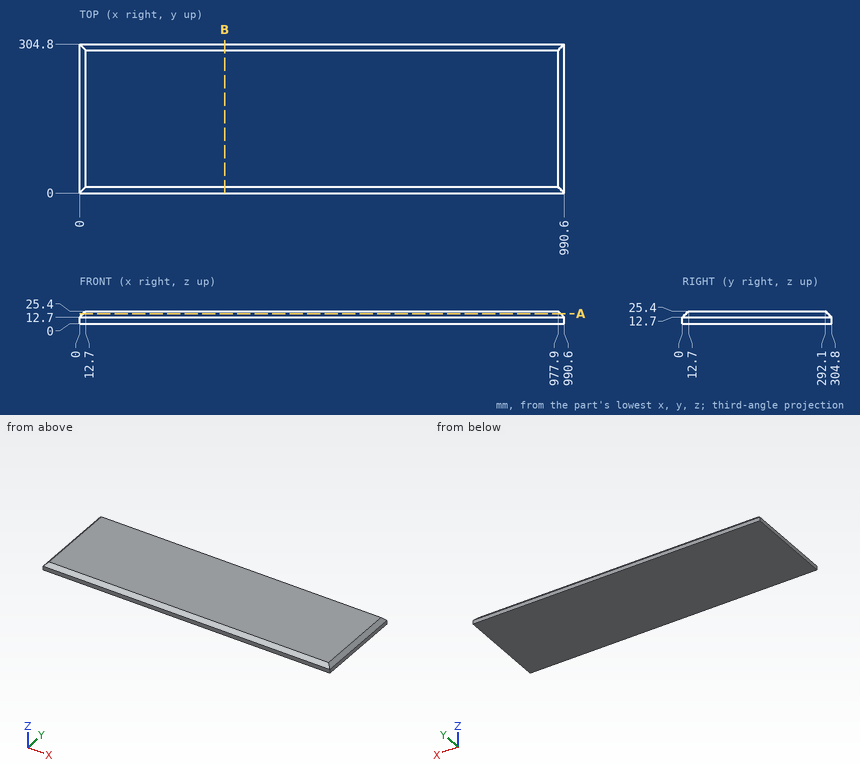
The drawing under review shows one solid part. Ordinate dimensions are in mm from its lowest x, y, z. Coordinates: 2 decimals unless noted, no trailing zeros. Write each loop counter-clockwise with the first axis right and the second up, starting at its lowest first coordinate (ties: lowest second). Pieces come first, ordered by that corner, then holes.
1) Add section A-A (z = 20.5). Write out the cut boundary in (x, y).
2) Insertion check: pin 1 (1 mm diameter, centred on y = 136.5, z = 21.5, fed in from +X). The pin has a flat end and moves straight along its axis. Give the tip position at first contact, or say it passes through.
3) Add section B-B (x = 296.5). Write out the cut boundary in (y, z).
4) To check wall thickness, follow L1, parallel to X at y = 67, z = 15; L2, parallel to X at y = 99, z = 15.5; L3, parallel to Y at x = 542, z = 16. State the ranges of each line that lie inside material, in increasing order.
Check result:
1. outline: (7.8, 7.8) - (982.8, 7.8) - (982.8, 297) - (7.8, 297) - close
2. pin 1: stops at x = 982.3
3. outline: (0, 0) - (304.8, 0) - (304.8, 12.7) - (292.1, 25.4) - (12.7, 25.4) - (0, 12.7) - close
4. L1: x = 2.3 to 988.3
4. L2: x = 2.8 to 987.8
4. L3: y = 3.3 to 301.5
